Verification items for this drawing (mm, ordinates from the low corner). Give positions to 0.01 mm unless a question says otherwise; leave off trailing zeros. Order: outer loops, then holes, each group sorted by start corner. A loop starts at its lowest first (then second) coordinate and runs counter-clockwise, first axis right, second up.
(1) Sectioned sample at B-B on z = 3.95. Record the cut outline in (x, y) (3 decimals).
(2) Gauge pin test, flat ends, axial feed: pin 1 (9 mm diameter, centred on x = 6.35, y = 12.5, fed in from +Z); pin 2 (4.5 mm diameter, centred on x = 135.5, y = 12, fed in from -Z). Record the tip position at first contact, or that the pin passes through.
(3) Scan lines: L1, parallel to X at y = 12.5, z = 0.5 (3 decimals); L2, parallel to X at y = 12.5, z = 3.9 (3 decimals); L3, parallel to Y at x = 6.35, z = 0.5. Record each from-to range of solid material in increasing order.
(4) Sectioned sample at A-A on x = 133.35. Record the cut outline in (y, z).
(5) Sectioned sample at C-C on y = 12.5. Record the cut outline in (x, z) (3 decimals).
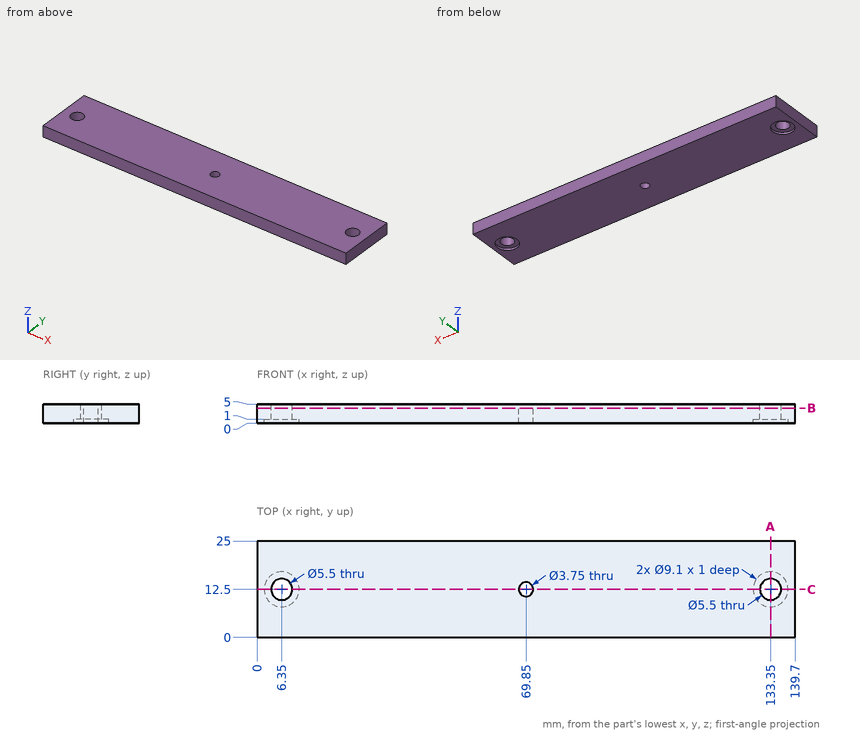
Ans:
1. outline: (0, 0) - (139.7, 0) - (139.7, 25) - (0, 25) - close; hole circle Ø5.5 at (6.35, 12.5); hole circle Ø3.75 at (69.85, 12.5); hole circle Ø5.5 at (133.35, 12.5)
2. pin 1: stops at z = 5
2. pin 2: stops at z = 1
3. L1: x = 0 to 1.8, 10.9 to 67.975, 71.725 to 128.8, 137.9 to 139.7
3. L2: x = 0 to 3.6, 9.1 to 67.975, 71.725 to 130.6, 136.1 to 139.7
3. L3: y = 0 to 7.95, 17.05 to 25
4. outline: (0, 0) - (7.95, 0) - (7.95, 1) - (9.75, 1) - (9.75, 5) - (0, 5) - close; (15.25, 1) - (17.05, 1) - (17.05, 0) - (25, 0) - (25, 5) - (15.25, 5) - close
5. outline: (0, 0) - (1.8, 0) - (1.8, 1) - (3.6, 1) - (3.6, 5) - (0, 5) - close; (9.1, 1) - (10.9, 1) - (10.9, 0) - (67.975, 0) - (67.975, 5) - (9.1, 5) - close; (71.725, 0) - (128.8, 0) - (128.8, 1) - (130.6, 1) - (130.6, 5) - (71.725, 5) - close; (136.1, 1) - (137.9, 1) - (137.9, 0) - (139.7, 0) - (139.7, 5) - (136.1, 5) - close
